Check sheet for the modelled part. Datum: model origin and axes. Units: mm. Give positions to 0.01 mm unless a question says otherwise; leave off trailing zeros. Loops run counter-clockwise (first coordinate to the right, second up) from the corner with the lowest first, then second, coordinate; pieces in that order, holes last. Notation, with made-up numbers: (4.5, 35.25) -> (38.5, 35.25) arc R27 ccw to (38.5, 53.25) -> close; hole circle Ø7 at (79.5, 82). An arc over 180 degrees is marked (long way). Write each question's results on one line, items separated by ' | '. Start each with the question number.
Item 1: Cross-section at A-A on x = -28. Enter the section's corners in (y, z), then the cut area to 3 significant figures.
Item 2: Cross-section at B-B on y = -24. Enter the section's corners in (x, z), then the cut area to 3 significant figures.
Item 3: Cross-section at C-C on z = 7.75. Enter the section's corners in (x, y).
Item 4: Scan lines: line 1 along X through (y, z) = (-24, 6.75); line 2 along Y through (x, z) = (28, 6.5). Record each from-to range of solid material in increasing order.
Item 5: Gauge pin test, flat end, axial feed: pin 1 Ø9 at (x, y) = (-28, -24) entering from -Z. Record the tip position at first contact, or that the pin passes through.
from build123d import *

# Parameters (mm, degrees)
SKETCH1_W           = 147
SKETCH1_H           = 137
SKETCH1_R           = 5.5
BOSS_EXTRUDE1_DEPTH = 9.25


with BuildPart() as part:
    # Sketch1 → Boss-Extrude1 (new body)
    with BuildSketch(Plane.XY.offset(9.25)):
        Rectangle(SKETCH1_W, SKETCH1_H)
        with Locations(Location((-28, -24, 0), (0, 0, 180))):
            Circle(SKETCH1_R, mode=Mode.SUBTRACT)
        with Locations(Location((28, -24, 0), (0, 0, 180))):
            Circle(SKETCH1_R, mode=Mode.SUBTRACT)
        with Locations(Location((28, 4, 0), (0, 0, 180))):
            Circle(SKETCH1_R, mode=Mode.SUBTRACT)
        with Locations(Location((-28, 4, 0), (0, 0, 180))):
            Circle(SKETCH1_R, mode=Mode.SUBTRACT)
    extrude(amount=-BOSS_EXTRUDE1_DEPTH)


solid = part.part
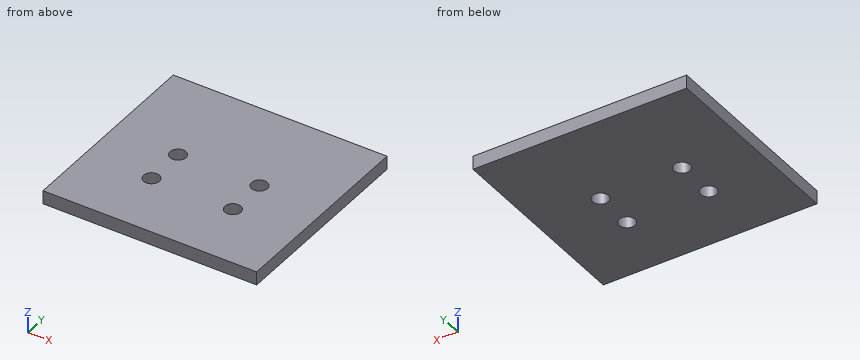
Answer sheet:
1) outline: (-68.5, 0) -> (-29.5, 0) -> (-29.5, 9.25) -> (-68.5, 9.25) -> close; (-18.5, 0) -> (-1.5, 0) -> (-1.5, 9.25) -> (-18.5, 9.25) -> close; (9.5, 0) -> (68.5, 0) -> (68.5, 9.25) -> (9.5, 9.25) -> close | area: 1,060 mm²
2) outline: (-73.5, 0) -> (-33.5, 0) -> (-33.5, 9.25) -> (-73.5, 9.25) -> close; (-22.5, 0) -> (22.5, 0) -> (22.5, 9.25) -> (-22.5, 9.25) -> close; (33.5, 0) -> (73.5, 0) -> (73.5, 9.25) -> (33.5, 9.25) -> close | area: 1,160 mm²
3) outline: (-73.5, -68.5) -> (73.5, -68.5) -> (73.5, 68.5) -> (-73.5, 68.5) -> close; hole circle Ø11 at (-28, -24); hole circle Ø11 at (-28, 4); hole circle Ø11 at (28, -24); hole circle Ø11 at (28, 4)
4) line 1: x = -73.5 to -33.5, -22.5 to 22.5, 33.5 to 73.5 | line 2: y = -68.5 to -29.5, -18.5 to -1.5, 9.5 to 68.5
5) pin 1: passes through
